The listing builds one solid part. Answer for the finished solid, in the listing's coordinates (mm). A direction names the side the tool comes from. Coordinates: 2 decimals unless noted, no trailing zeros. Order: outer loops, then holes, each group sorted by start corner. A loop starts at its lowest first (then second) coordinate and runs counter-clockwise, first axis right, second up.
```python
from build123d import *

# Parameters (mm, degrees)
F1_DEPTH = 5.334
F2_DEPTH = 5.334
F4_DEPTH = 5.334


with BuildPart() as f1:
    # F0 (on Front) → F1 (new body)
    with BuildSketch(Plane.XZ):
        with BuildLine():
            ThreePointArc((27.324475, 0), (19.600425, -19.741603), (0, -27.817197))
            ThreePointArc((0, -27.817197), (62.043611, -61.433), (27.324475, 0))
        make_face()
    extrude(amount=F1_DEPTH)

    # F1_face (on face) → F2 (join)
    with BuildSketch(Plane(origin=(37.914112, -5.334, -37.730903), x_dir=(1, 0, 0), z_dir=(0, -1, 0))):
        with BuildLine():
            ThreePointArc((-10.589637, 37.730903), (-18.313687, 17.9893), (-37.914112, 9.913706))
            ThreePointArc((-37.914112, 9.913706), (24.129499, -23.702097), (-10.589637, 37.730903))
        make_face()
    extrude(amount=F2_DEPTH)

    # F3 (on face) → F4 (join)
    with BuildSketch(Plane.XZ.offset(10.668)):
        Polygon((47.816351, -34.752887), (27.324475, -35.03488), (27.324475, -40.946536), (40.31878, -40.946536), (35.429053, -56.267668), (40.31878, -56.267668), align=None)
        Polygon((21.411845, -34.752887), (14.236325, -35.03488), (14.236325, -56.267668), (21.411845, -56.267668), align=None)
    extrude(amount=F4_DEPTH)


solid = f1.part
```
1) A cutting plane is placed at D-D, the plane y = -2. Write down the section's boundary in (x, z).
2) Straight lines are drawn through the part: probe 1 along Y at (x, z) = (20, -56.5); probe 2 along X at (y, z) = (-1.75, -14.5); probe 3 along X at (y, z) = (-4.5, -45.5) (3 decimals). For each, find the intervals that lie inside material, in ascending order.
3) Each of these flat-tipped pins is pushed along its axis until it touches: P1, Ø2.5, axis at x = 18, y = -12, coming from the -Z side; P2, Ø3, axis at x = 29, z = -57, coming from the -Y side; P3, Ø2.5, axis at y = -12, z = -39.5, coming from the -X side. Where does it stop, or does it pass through?
4) A cutting plane is placed at C-C, the plane z = -45. Write down the section's boundary in (x, y), plus the area to 3 significant figures.
5) A cutting plane is placed at A-A, the plane y = -12.5. Write down the section's boundary in (x, z).
6) The mould has two halves that part along X. Classify faces 1 (the flat face through (37.4, -16.002, -40.6)), 2 (the cylindrical face through (61.1, -5.26, -62.36)), 3 (the flat face through (37.91, -13.3, -48.5)): released by +X, released by -X, zero draft, split by the parting line, or undercut.
7) A cutting plane is placed at B-B, the plane x = 28.5. Write down the section's boundary in (y, z).
8) For faces 4 (the flat face through (27.324, -13, -38)), 5 (the flat face through (17.874, -13.298, -34.892)), 6 (the flat face through (18, -13, -56.268)), 7 (the flat face through (44, -13.3, -45.7)), determine the directions among +Z, -Z, +X, -X, +Y, -Y from which every point of the face is accessible in a straight line to the end or side of a thin tool.
Working result:
1. outline: (0, -27.82) arc R36.71 ccw (long way) to (27.32, 0) arc R26.99 cw to start
2. probe 1: y = -10.67 to 0
2. probe 2: x = 23.62 to 65.82
2. probe 3: x = 0.472 to 71.235
3. P1: stops at z = -56.27
3. P2: stops at y = -10.67
3. P3: stops at x = 14.24
4. outline: (0.34, -10.67) - (14.24, -10.67) - (14.24, -16) - (21.41, -16) - (21.41, -10.67) - (39.03, -10.67) - (39.03, -16) - (44.25, -16) - (44.25, -10.67) - (71.37, -10.67) - (71.37, 0) - (0.34, 0) - close
4. area: 824 mm2
5. outline: (14.24, -56.27) - (21.41, -56.27) - (21.41, -34.75) - (14.24, -35.03) - close; (27.32, -40.95) - (40.32, -40.95) - (35.43, -56.27) - (40.32, -56.27) - (47.82, -34.75) - (27.32, -35.03) - close
6. face 1: zero draft
6. face 2: split by the parting line
6. face 3: undercut
7. outline: (-16, -40.95) - (-10.67, -40.95) - (-10.67, -71.67) - (0, -71.67) - (0, 0.26) - (-10.67, 0.26) - (-10.67, -35.02) - (-16, -35.02) - close
8. face 4: +Z, -Z, -Y
8. face 5: +Z, -X, -Y
8. face 6: -Z, +X, -X, -Y
8. face 7: -Z, +X, -Y
